Design review of the part built by this model. Coordinates are the model's own, in mm. Coordinates: 2 decimals unless noted, no trailing zeros. Loops run counter-clockwise (first coordinate to the right, second up) from the corner with the lowest first, then second, coordinate; pieces in that order, holes last. Notation, with made-up numbers: M -13.75,-33 L -0.75,-33 A27 ccw -0.75,-14 Z; hole C -8,86 d5. An arc over 180 degrees is marked long. One line per item, written item: value.
```python
from build123d import *

# Parameters (mm, degrees)
SKETCH_1_R                   = 100
EXTRUDE_1_DEPTH              = 5
HOLE_WIZARD_M3_1_D           = 2.5
HOLE_WIZARD_M3_1_CSINK_D     = 9.05
HOLE_WIZARD_M3_1_CSINK_ANGLE = 90
SKETCH_5_R                   = 12.5
CUT_EXTRUDE_1_DEPTH          = 142.509716981
HOLE_WIZARD_M4_2_D           = 3.3
HOLE_WIZARD_M4_2_DEPTH       = 5
HOLE_WIZARD_M4_2_CSINK_D     = 4.05
HOLE_WIZARD_M4_2_CSINK_ANGLE = 90


with BuildPart() as part:
    # 草图1 → 凸台-拉伸1 (new body)
    with BuildSketch(Plane(origin=(0, 0, 0), x_dir=(1, 0, 0), z_dir=(0, 1, 0))):
        with Locations(Location((0, 0, 0), (0, 0, 270))):
            Circle(SKETCH_1_R)
    extrude(amount=EXTRUDE_1_DEPTH)

    # M3 螺纹孔1 (through all)
    with Locations(Plane(origin=(0, 5, 0), x_dir=(1, 0, 0), z_dir=(0, 1, 0))):
        with Locations((0, 20), (17.320508076, -10), (-17.320508076, -10)):
            CounterSinkHole(HOLE_WIZARD_M3_1_D / 2, HOLE_WIZARD_M3_1_CSINK_D / 2, counter_sink_angle=HOLE_WIZARD_M3_1_CSINK_ANGLE)

    # 草图5 → 切除-拉伸1 (cut, through all)
    with BuildSketch(Plane(origin=(0, 5, 0), x_dir=(1, 0, 0), z_dir=(0, 1, 0))):
        with Locations(Location((0, 0, 0), (0, 0, 270))):
            Circle(SKETCH_5_R)
    extrude(amount=-CUT_EXTRUDE_1_DEPTH, mode=Mode.SUBTRACT)

    # M4 螺纹孔2
    with Locations(Plane(origin=(0, 5, 0), x_dir=(1, 0, 0), z_dir=(0, 1, 0))):
        with Locations((0, 0), (-28.35, 85), (28.35, 85), (28.35, -85), (-28.35, -85), (-28.35, 60), (28.35, 60), (-28.35, -60), (28.35, -60)):
            CounterSinkHole(HOLE_WIZARD_M4_2_D / 2, HOLE_WIZARD_M4_2_CSINK_D / 2, depth=HOLE_WIZARD_M4_2_DEPTH, counter_sink_angle=HOLE_WIZARD_M4_2_CSINK_ANGLE)


solid = part.part
```
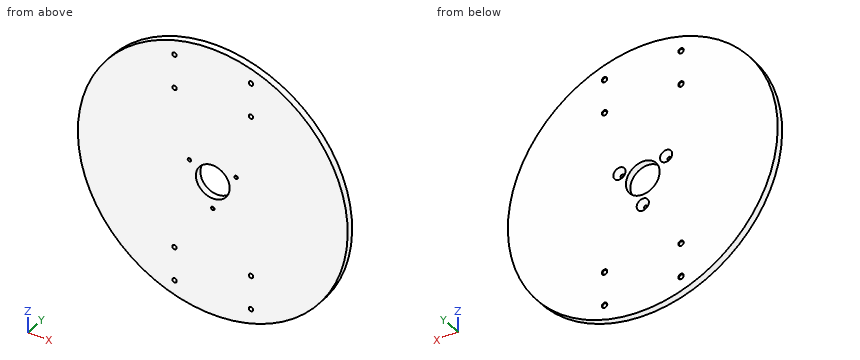
(1) We need section C-C on y = 3.1. State how many separate pieces and enclosed holes the cut face has, then the cut area to 3 significant figures.
Reply:
separate pieces: 1
enclosed holes: 12
area: 30,800 mm2
(2) We need section A-A on z = 0. State the section outline as (x, y) points, then the cut area to 3 significant figures.
Reply:
outline: M -100,0 L -12.5,0 L -12.5,5 L -100,5 Z; M 12.5,0 L 100,0 L 100,5 L 12.5,5 Z
area: 875 mm2
(3) We need section B-B on x = -9. State the section outline as (y, z) points, then the cut area to 3 significant figures.
Reply:
outline: M 0,-99.59 L 5,-99.59 L 5,-8.67 L 0,-8.67 Z; M 0,8.67 L 5,8.67 L 5,99.59 L 0,99.59 Z
area: 909 mm2
(4) To check wall thickness, follow line 1 along X through (y, z) = (3.5, 60); line 2 along X through (y, z) = (2.9, -85); line 3 along Z through (x, y) = (-28.35, 2.1). State the ranges of each line that lie inside material, in increasing order. Write a range as [from, to].
Reply:
line 1: x = [-80, -30], [-26.7, 26.7], [30, 80]
line 2: x = [-52.68, -30], [-26.7, 26.7], [30, 52.68]
line 3: z = [-95.9, -86.65], [-83.35, -61.65], [-58.35, 58.35], [61.65, 83.35], [86.65, 95.9]
(5) Insertion check: pin 1 (1 mm diameter, centred on y = 3, z = -36, fed in from +X); pin 2 (1.5 mm diameter, centred on x = 21, y = 0.5, fed in from -Z); pin 3 (4 mm diameter, centred on x = 28.35, z = -60, fed in from +Y) (3 decimals); pin 4 (3 mm diameter, centred on x = -28.35, z = 60, fed in from -Y). Each pin has a flat end and moves straight along its axis. Give the tip position at first contact, or say it passes through.
Reply:
pin 1: stops at x = 93.49
pin 2: stops at z = -97.93
pin 3: stops at y = 4.975
pin 4: passes through
(6) We need section D-D on x = -68.5. State the section outline as (y, z) points, then the cut area to 3 significant figures.
Reply:
outline: M 0,-72.85 L 5,-72.85 L 5,72.85 L 0,72.85 Z
area: 729 mm2
